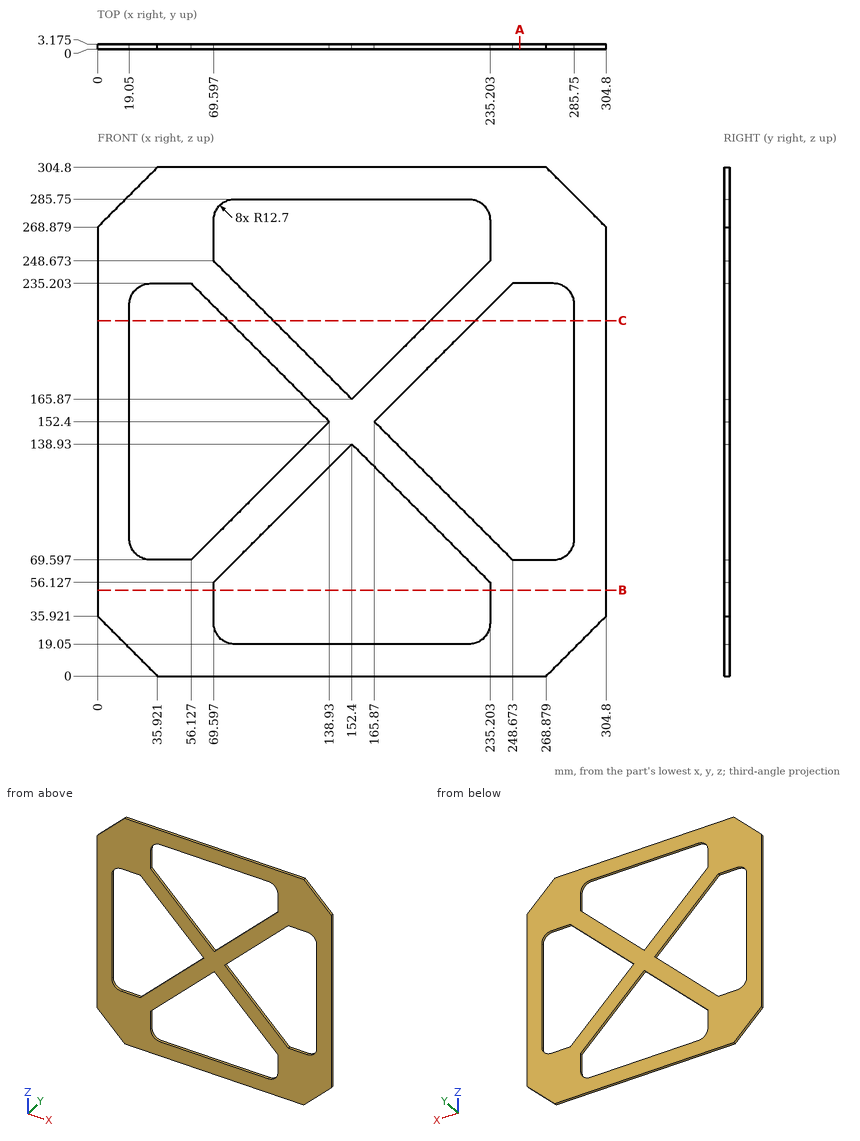
The figure shows three views and two pictorial views of one solid part (mm, origin at its lowest corner). Answer the questions. Give positions to 0.01 mm unless a question says otherwise; leave off trailing zeros. Write each loop counter-clockwise with the first axis right and the second up, starting at its lowest first coordinate (ties: lowest second). Pieces come first, ordered by that corner, then holes.
Q1. The part is cut by section A-A on x = 253. Give the vertices of the cut face in (y, z) (1 decimal).
Answer:
outline: (0, 0) - (3.2, 0) - (3.2, 69.6) - (0, 69.6) - close; (0, 235.2) - (3.2, 235.2) - (3.2, 304.8) - (0, 304.8) - close
Q2. The part is cut by section C-C on z = 213. State how many separate pieces and enclosed holes the cut face has, and give its area (3 significant figures).
Answer:
separate pieces: 4
enclosed holes: 0
area: 292 mm2
Q3. Given pin 1 (1.6 mm diameter, centred on y = 1.5, z = 40, fed in from -X), flat-ended and moving along its own axis, determine where the tip first touches the part or whether it passes through.
Answer:
pin 1: stops at x = 0
Q4. The part is cut by section B-B on z = 51.5. Give the vertices of the cut face in (x, y) (1 decimal), and give its area (3 significant figures).
Answer:
outline: (0, 0) - (69.6, 0) - (69.6, 3.2) - (0, 3.2) - close; (235.2, 0) - (304.8, 0) - (304.8, 3.2) - (235.2, 3.2) - close
area: 442 mm2
Q5. Straight lines are drawn through the part: L1, parallel to X at y = 2.5, z = 48; L2, parallel to X at y = 2.9, z = 162.5; L3, parallel to Z at x = 104.5, y = 1.15. For each, find the intervals that lie inside material, in ascending order.
Answer:
L1: x = 0 to 69.6, 235.2 to 304.8
L2: x = 0 to 19.05, 128.83 to 175.97, 285.75 to 304.8
L3: z = 0 to 19.05, 91.03 to 117.97, 186.83 to 213.77, 285.75 to 304.8
